The model under review builds one solid part; all positions refer to its coordinate system, in mm. Face numbers are marked on the shaded views. Coordinates: 2 decimals unless noted, no trailing zeros. Order: outer loops, then holes, each group sorted by start corner. A loop starts at its lowest first (then second) coordinate and runs counter-clockwise, first axis right, second up. Notation, with made-up numbers: M 35.25,-30.75 L 79.25,-30.75 A10 ccw 79.25,-20.75 Z; hole C 65,24.5 d10. An arc over 180 degrees is marked long. One line per item, written item: value.
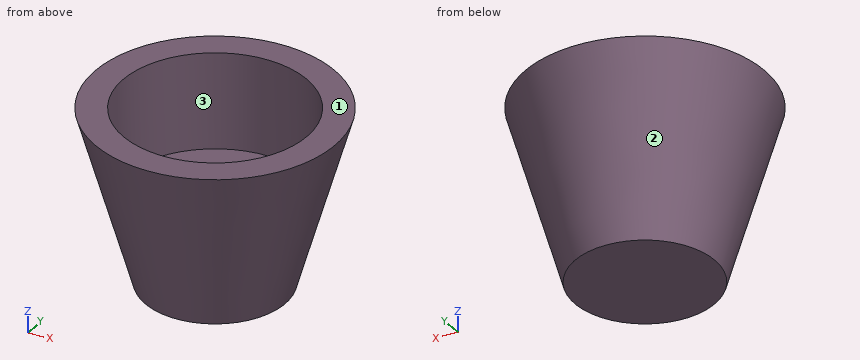
```python
from build123d import *

# Parameters (mm, degrees)
F2_R     = 24.421659
F3_DEPTH = 25.4
F4_R     = 12.060942
F5_DEPTH = 18.542


with BuildPart() as f1:
    # F0 (on Front) → F1 (revolve)
    with BuildSketch(Plane.XZ):
        Polygon((0, -26.049769), (0, 20.002501), (-31.864449, 20.002501), (-18.606978, -26.049769), align=None)
    revolve(axis=Axis((0, 0, -3.023634), (0, 0, -1)))

    # F2 (on face) → F3 (cut)
    with BuildSketch(Plane.XY.offset(20.002501)):
        Circle(F2_R)
    extrude(amount=-F3_DEPTH, mode=Mode.SUBTRACT)

    # F4 (on face) → F5 (cut)
    with BuildSketch(Plane.XY.offset(-5.397499)):
        Circle(F4_R)
    extrude(amount=-F5_DEPTH, mode=Mode.SUBTRACT)


solid = f1.part
```
(1) Mouldability with a two-part tool opening along X and no side actions: class the marked faces 1, 2 and 3 as +X half, -X half, draft (parallel to the pull), parting line (faces both ways), or undercut.
Geometry results:
face 1: draft
face 2: parting line
face 3: undercut
(2) Insertion check: pin 1 Ø1 at (y, z) = (-10, 7) entering from -X; pin 2 Ø2 at (x, y) = (9, -11) entering from +Z; pin 3 Ø1.5 at (y, z) = (18, -7) entering from -X. Each pin has a flat end and moves straight along its axis. Give the tip position at first contact, or say it passes through.
Geometry results:
pin 1: stops at x = -26.52
pin 2: stops at z = -5.4
pin 3: stops at x = -16.88
(3) We need section C-C, the plane z = 6.5. State the section outline as (x, y) points, plus the area to 3 significant figures.
Geometry results:
outline: C 0,0 d55.95; hole C 0,0 d48.84
area: 585 mm2
(4) We need section A-A, the plane y = 0. State the section outline as (x, z) points, plus the area to 3 significant figures.
Geometry results:
outline: M -31.86,20 L -18.61,-26.05 L 18.61,-26.05 L 31.86,20 L 24.42,20 L 24.42,-5.4 L 12.06,-5.4 L 12.06,-23.94 L -12.06,-23.94 L -12.06,-5.4 L -24.42,-5.4 L -24.42,20 Z
area: 636 mm2
(5) We need section D-D, the plane z = 0.5. State the section outline as (x, y) points.
Geometry results:
outline: C 0,0 d52.5; hole C 0,0 d48.84
(6) For L1, parallel to Z at x = -9, y = -8.5; L2, parallel to Z at x = -0.5, y = -8.5; L3, parallel to Y at x = 0, z = -14, list the stretches that pass through material, from the lowest coordinate up.
Geometry results:
L1: z = -26.05 to -5.4
L2: z = -26.05 to -23.94
L3: y = -22.08 to -12.06, 12.06 to 22.08
